Could you check a few things on this model? Use its own coordinates, in mm. Coordinates: 2 decimals unless noted, no trailing zeros. Order: outer loops, then holes, each group sorted by start corner. A loop starts at its lowest first (then second) coordinate and runs counter-clockwise, first axis right, second up.
```python
from build123d import *

# Parameters (mm, degrees)
F0_W     = 38.1
F0_H     = 38.1
F1_DEPTH = 101.6
F2_SIZE  = 6.35
F4_D     = 17.4625
F5_D     = 4.7625


with BuildPart() as f1:
    # F0 (on Front) → F1 (new body)
    with BuildSketch(Plane.XZ):
        Rectangle(F0_W, F0_H)
    extrude(amount=-F1_DEPTH)

    # F2
    f2_edges = [f1.edges().sort_by_distance(p)[0] for p in [
        (19.05, 101.6, 0),
    ]]
    chamfer(f2_edges, length=F2_SIZE)

    # F4 (through all)
    with Locations(Plane.YZ.offset(19.05)):
        with Locations((50.8, 0)):
            Hole(F4_D / 2)

    # F5 (through all)
    with Locations(Plane.YZ.offset(19.05)):
        with Locations((15.875, 0), (85.725, 0)):
            Hole(F5_D / 2)


solid = f1.part
```
Item 1: I need wall thicknesses on line 1 (Y direction, x = -16.5, z = 2); line 2 (Z direction, x = -15, y = 56.5); line 3 (Z direction, x = -6, y = 50.8). Which ranges of each line are inside material? Lowest first, please.
Item 2: Suppose I cut it at A-A (y = 50.8). List the corners of the cut face in (x, z) for me.
Item 3: For pin 1 Ø2 at (x, z) = (-12, 9.5) entering from -Y; pin 2 Ø4.5 at (y, z) = (15.875, 0) entering from -X, each with a flat end and sliding along its axis, tell me the tip position at first contact or that it passes through.
Item 4: Suppose I cut it at C-C (x = 14.5). Count the separate pieces of the cut face and the enclosed holes in it, and give its area (3 significant figures).
Item 5: Thinking about a two-plate mould opening in Z: for faces 1 (the face through (0, 0, 0)), 2 (the face through (-0.3, 13.6, 0.7)), 3 (the face through (0, 50, -19.05)), which applies, +Z half, -Z half, draft (parallel to the pull), parting line (faces both ways), or undercut?
Item 6: Suppose I cut it at D-D (z = -7). List the corners of the cut face in (x, y) for me, and give its area (3 significant figures).
Item 7: Suppose I cut it at B-B (z = 0). List the corners of the cut face in (x, y) for me, and give its area (3 significant figures).
Geometry results:
1. line 1: y = 0 to 14.58, 17.17 to 42.3, 59.3 to 84.43, 87.02 to 101.6
1. line 2: z = -19.05 to -6.61, 6.61 to 19.05
1. line 3: z = -19.05 to -8.73, 8.73 to 19.05
2. outline: (-19.05, -19.05) - (19.05, -19.05) - (19.05, -8.73) - (-19.05, -8.73) - close; (-19.05, 8.73) - (19.05, 8.73) - (19.05, 19.05) - (-19.05, 19.05) - close
3. pin 1: stops at y = 0
3. pin 2: passes through
4. separate pieces: 1
4. enclosed holes: 3
4. area: 3,530 mm2
5. face 1: draft
5. face 2: undercut
5. face 3: -Z half
6. outline: (-19.05, 0) - (19.05, 0) - (19.05, 45.58) - (-19.05, 45.58) - close; (-19.05, 56.02) - (19.05, 56.02) - (19.05, 95.25) - (12.7, 101.6) - (-19.05, 101.6) - close
6. area: 3,450 mm2
7. outline: (-19.05, 0) - (19.05, 0) - (19.05, 13.49) - (-19.05, 13.49) - close; (-19.05, 18.26) - (19.05, 18.26) - (19.05, 42.07) - (-19.05, 42.07) - close; (-19.05, 59.53) - (19.05, 59.53) - (19.05, 83.34) - (-19.05, 83.34) - close; (-19.05, 88.11) - (19.05, 88.11) - (19.05, 95.25) - (12.7, 101.6) - (-19.05, 101.6) - close
7. area: 2,820 mm2
